```python
from build123d import *

# Parameters (mm, degrees)
SKETCH1_R           = 4.25
BOSS_EXTRUDE1_DEPTH = 5
CUT_EXTRUDE1_DEPTH  = 3
FILLET1_R           = 0.5


with BuildPart() as part:
    # Sketch1 → Boss-Extrude1 (new body)
    with BuildSketch(Plane(origin=(0, 0, 0), x_dir=(1, 0, 0), z_dir=(0, 1, 0))):
        Circle(SKETCH1_R)
    extrude(amount=BOSS_EXTRUDE1_DEPTH)

    # Sketch2 → Cut-Extrude1 (cut)
    with BuildSketch(Plane(origin=(0, 5, 0), x_dir=(1, 0, 0), z_dir=(0, 1, 0))):
        Polygon((-2.309401077, 0), (-1.154700538, -2), (1.154700538, -2), (2.309401077, 0), (1.154700538, 2), (-1.154700538, 2), align=None)
    extrude(amount=-CUT_EXTRUDE1_DEPTH, mode=Mode.SUBTRACT)

    # Fillet1
    fillet1_edges = [part.edges().sort_by_distance(p)[0] for p in [
        (-4.25, 5, 0),
    ]]
    fillet(fillet1_edges, radius=FILLET1_R)


solid = part.part
```
CAD build for the part. Positions are in the model's coordinates, mm. A direction names the side the tool comes from. Give positions to 0.01 mm unless a question says otherwise; leave off trailing zeros. Order: outer loops, then holes, each group sorted by start corner. A loop starts at its lowest first (then second) coordinate and runs counter-clockwise, first axis right, second up. Notation, with made-up numbers: M 15,-15.75 L 57,-15.75 A18 ccw 57,16.25 Z; hole C 72,73 d8. An arc over 180 degrees is marked long. Put each result on its own line as item: value. Start each with the question number.
(1) Flat gauge pins, fed straight in: pin 1 Ø1.5 at (x, y) = (-2, 4) entering from -Z; pin 2 Ø0.7 at (x, y) = (-0.5, 3.5) entering from -Z. Where does each tip first touch, or does it go through?
(2) Saw through at C-C, the plane y = 1.1. Write the cut outline in (x, z).
(3) Which spindle directions (+Z, -Z, +X, -X, +Y, -Y) get a long thin tool onto all of the face, cutting with end or side? Do faces 1 (the flat face through (0, 4, -2)), 2 (the flat face through (2, 5, 2)). Say none if no direction does.
(4) Drill centre lines: line 1 along Z through (x, y) = (-3.75, 2.95); line 2 along X through (y, z) = (2.15, -0.25); line 3 along Y through (x, z) = (-2, 0.25). Where is each one in solid material? Low to high.
(5) Mould opens along Z. For faces 3 (the flat face through (0, 0, 0)), 4 (the cylindrical face through (2.285, 2.218, -3.584)), 5 (the flat face through (0, 4, 2)) say: +Z half, -Z half, draft (parallel to the pull), parting line (faces both ways), or undercut.
(6) Saw through at A-A, the plane y = 2.7. Write the cut outline in (x, z), then the cut area to 3 significant figures.
(7) Saw through at B-B, the plane x = 0. Write the cut outline in (y, z).
Check result:
1. pin 1: stops at z = -4.06
1. pin 2: stops at z = -4.25
2. outline: C 0,0 d8.5
3. face 1: +Y
3. face 2: +Z, -Z, +X, -X, +Y
4. line 1: z = -2 to 2
4. line 2: x = -4.24 to -2.17, 2.17 to 4.24
4. line 3: y = 0 to 2
5. face 3: draft
5. face 4: parting line
5. face 5: undercut
6. outline: C 0,0 d8.5; hole M -2.31,0 L -1.15,-2 L 1.15,-2 L 2.31,0 L 1.15,2 L -1.15,2 Z
6. area: 42.9 mm2
7. outline: M 0,-4.25 L 4.5,-4.25 A0.5 ccw 5,-3.75 L 5,-2 L 2,-2 L 2,2 L 5,2 L 5,3.75 A0.5 ccw 4.5,4.25 L 0,4.25 Z
